For this review, take the finished solid that the model builds, in its own axes (mm). A direction names the side the tool comes from. Give positions to 0.01 mm unless a question says otherwise; leave off trailing zeros. Write each loop counter-clockwise with the first axis right and the second up, starting at its lowest first coordinate (ties: lowest second). Pieces come first, ordered by that corner, then holes.
Q1. Mouldability with a two-part tool opening along X and no side actions: class faces 3 (the cylindrical face through (90.047, -9.33, 29.268)), 4 (the cylindrical face through (140.345, -8.762, 50.263)), 5 (the flat face through (79, -9, 57.15)), 6 (the flat face through (70.353, -9.392, 10.776)) as released by +X, released by -X, zero draft, split by the parting line, or undercut.
Q2. We need section B-B (z = 39.5). Write out the cut boundary in (x, y) (3 decimals), then the cut area to 3 significant figures.
Q3. For line 1 (X direction, y = -9.75, z = 50); line 2 (X direction, y = -11.75, z = 45); line 3 (X direction, y = -13.5, z = 34.5), list the stretches that pass through material, from the lowest coordinate up.
Q4. We need section C-C (x = 95). Write out the cut boundary in (y, z), then the cut area to 3 significant figures.
Q5. We need section D-D (x = 125). Write out the cut boundary in (y, z).
Q6. We need section A-A (x = 50.8). Write out the cut boundary in (y, z) (3 decimals).
Q7. Insertion check: P1, Ø10, axis at x = 137.922, y = -9.525, coming from the -Z side; P2, Ø10, axis at x = 94.5, y = -11.5, coming from the -Z side; P3, Ø6, axis at x = 94.488, y = -9.525, coming from the -Z side. Each pin has a flat end and moves straight along its axis. Give the tip position at first contact, or say it passes through.
Q8. Machinability: for faces 1 (the cylindrical face through (133.48, -9.33, 39.6)), 2 (the flat face through (120.365, -9.392, 28.061)), which of the approach directions +Z, -Z, +X, -X, +Y, -Y give a long, thin tool a straight path to every point of the face, cutting with its end or side? Answer none if there is none.
```python
from build123d import *

# Parameters (mm, degrees)
F1_DEPTH  = 19.05
F2_R      = 2.54
F3_DEPTH  = 50.801
F4_START  = -13.97
F2_R_2    = 4.445
F4_DEPTH  = 40.386
F6_DEPTH  = 10.16
F8_DEPTH  = 10.16
F10_DEPTH = 10.16


with BuildPart() as f1:
    # F0 (on Front) → F1 (new body)
    with BuildSketch(Plane.XZ):
        Polygon((149.77654996, 57.15), (6.35, 57.15), (6.35, 6.35), (49.53, 6.35), (91.7664133997, 15.3276268095), (149.77654996, 41.1554036448), align=None)
    extrude(amount=F1_DEPTH)

    # F2 (on face) → F3 (cut, through all)
    with BuildSketch(Plane.XY.offset(57.15)):
        with Locations((50.8, -9.525)):
            Circle(F2_R)
        with Locations((94.488, -9.525)):
            Circle(F2_R)
        with Locations((137.922, -9.525)):
            Circle(F2_R)
    extrude(amount=-F3_DEPTH, mode=Mode.SUBTRACT)

    # F2 (on face) → F4 (cut)
    with BuildSketch(Plane.XY.offset(57.15).offset(F4_START)):
        with Locations((50.8, -9.525)):
            Circle(F2_R_2)
        with Locations((50.8, -9.525)):
            Circle(F2_R, mode=Mode.SUBTRACT)
        with Locations((94.488, -9.525)):
            Circle(F2_R_2)
        with Locations((94.488, -9.525)):
            Circle(F2_R, mode=Mode.SUBTRACT)
        with Locations((137.922, -9.525)):
            Circle(F2_R_2)
        with Locations((137.922, -9.525)):
            Circle(F2_R, mode=Mode.SUBTRACT)
    extrude(amount=-F4_DEPTH, mode=Mode.SUBTRACT)

    # F5 (on face) → F6 (cut)
    with BuildSketch(Plane(origin=(0, 0, 6.35), x_dir=(1, 0, 0), z_dir=(0, 0, -1))):
        with BuildLine():
            ThreePointArc((21.0968814449, 14.0652501177), (20.97463405, 14.5484294642), (20.6373100259, 14.915334369))
            ThreePointArc((20.6373100259, 14.915334369), (20.0808814449, 14.0652501177), (19.6229011784, 13.1583267056))
            ThreePointArc((19.6229011784, 13.1583267056), (20.6133042324, 13.1999282265), (21.0968814449, 14.0652501177))
        make_face()
        with BuildLine():
            ThreePointArc((19.6229011784, 13.1583267056), (20.0808814449, 14.0652501177), (20.6373100259, 14.915334369))
            ThreePointArc((20.6373100259, 14.915334369), (19.2009996347, 14.5732501177), (19.6229011784, 13.1583267056))
        make_face()
        with BuildLine():
            ThreePointArc((36.8247688031, 4.9847501177), (36.6740906943, 5.5171729052), (36.2667490696, 5.8916735299))
            ThreePointArc((36.2667490696, 5.8916735299), (35.8087688031, 4.9847501177), (35.2523402221, 4.1346658664))
            ThreePointArc((35.2523402221, 4.1346658664), (36.2919481496, 4.0909975126), (36.8247688031, 4.9847501177))
        make_face()
        with BuildLine():
            ThreePointArc((35.2523402221, 4.1346658664), (35.8087688031, 4.9847501177), (36.2667490696, 5.8916735299))
            ThreePointArc((36.2667490696, 5.8916735299), (34.9288869928, 5.4927501177), (35.2523402221, 4.1346658664))
        make_face()
    extrude(amount=-F6_DEPTH, mode=Mode.SUBTRACT)

    # F7 (on face) → F8 (cut)
    with BuildSketch(Plane(origin=(0.8496578997, 0, -3.9973261378), x_dir=(0.9781476007, 0, 0.2079116908), z_dir=(0.2079116908, 0, -0.9781476007))):
        with BuildLine():
            ThreePointArc((64.5139077337, 14.0652501177), (64.3916603388, 14.5484294642), (64.0543363147, 14.915334369))
            ThreePointArc((64.0543363147, 14.915334369), (63.4979077337, 14.0652501177), (63.0399274672, 13.1583267056))
            ThreePointArc((63.0399274672, 13.1583267056), (64.0303305212, 13.1999282265), (64.5139077337, 14.0652501177))
        make_face()
        with BuildLine():
            ThreePointArc((63.0399274672, 13.1583267056), (63.4979077337, 14.0652501177), (64.0543363147, 14.915334369))
            ThreePointArc((64.0543363147, 14.915334369), (62.6180259235, 14.5732501177), (63.0399274672, 13.1583267056))
        make_face()
        with BuildLine():
            ThreePointArc((80.2417950919, 4.9847501177), (80.0911169831, 5.5171729052), (79.6837753584, 5.8916735299))
            ThreePointArc((79.6837753584, 5.8916735299), (79.2257950919, 4.9847501177), (78.6693665109, 4.1346658664))
            ThreePointArc((78.6693665109, 4.1346658664), (79.7089744384, 4.0909975126), (80.2417950919, 4.9847501177))
        make_face()
        with BuildLine():
            ThreePointArc((78.6693665109, 4.1346658664), (79.2257950919, 4.9847501177), (79.6837753584, 5.8916735299))
            ThreePointArc((79.6837753584, 5.8916735299), (78.3459132816, 5.4927501177), (78.6693665109, 4.1346658664))
        make_face()
    extrude(amount=-F8_DEPTH, mode=Mode.SUBTRACT)

    # F9 (on face) → F10 (cut)
    with BuildSketch(Plane(origin=(9.4860255039, 0, -21.30596212), x_dir=(0.9135454576, 0, 0.4067366431), z_dir=(0.4067366431, 0, -0.9135454576))):
        with BuildLine():
            ThreePointArc((105.3219744595, 14.06525), (105.1997270646, 14.5484293465), (104.8624030404, 14.9153342513))
            ThreePointArc((104.8624030404, 14.9153342513), (104.3059744595, 14.06525), (103.847994193, 13.1583265879))
            ThreePointArc((103.847994193, 13.1583265879), (104.8383972469, 13.1999281088), (105.3219744595, 14.06525))
        make_face()
        with BuildLine():
            ThreePointArc((103.847994193, 13.1583265879), (104.3059744595, 14.06525), (104.8624030404, 14.9153342513))
            ThreePointArc((104.8624030404, 14.9153342513), (103.4260926492, 14.57325), (103.847994193, 13.1583265879))
        make_face()
        with BuildLine():
            ThreePointArc((121.0498618176, 4.98475), (120.8991837088, 5.5171727875), (120.4918420841, 5.8916734121))
            ThreePointArc((120.4918420841, 5.8916734121), (120.0338618176, 4.98475), (119.4774332367, 4.1346657487))
            ThreePointArc((119.4774332367, 4.1346657487), (120.5170411641, 4.0909973949), (121.0498618176, 4.98475))
        make_face()
        with BuildLine():
            ThreePointArc((119.4774332367, 4.1346657487), (120.0338618176, 4.98475), (120.4918420841, 5.8916734121))
            ThreePointArc((120.4918420841, 5.8916734121), (119.1539800074, 5.49275), (119.4774332367, 4.1346657487))
        make_face()
    extrude(amount=-F10_DEPTH, mode=Mode.SUBTRACT)


solid = f1.part
```
Computed:
1. face 3: undercut
1. face 4: undercut
1. face 5: zero draft
1. face 6: released by +X
2. outline: (6.35, -19.05) - (146.058, -19.05) - (146.058, 0) - (6.35, 0) - close; hole circle Ø8.89 at (50.8, -9.525); hole circle Ø8.89 at (94.488, -9.525); hole circle Ø8.89 at (137.922, -9.525)
2. area: 2,480 mm2
3. line 1: x = 6.35 to 48.27, 53.33 to 91.96, 97.02 to 135.39, 140.45 to 149.78
3. line 2: x = 6.35 to 49.57, 52.03 to 93.26, 95.71 to 136.7, 139.15 to 149.78
3. line 3: x = 6.35 to 48.81, 52.79 to 92.5, 96.48 to 134.83
4. outline: (-19.05, 16.77) - (-13.94, 16.77) - (-13.94, 43.18) - (-12.01, 43.18) - (-12.01, 57.15) - (-19.05, 57.15) - close; (-7.04, 43.18) - (-5.11, 43.18) - (-5.11, 16.77) - (0, 16.77) - (0, 57.15) - (-7.04, 57.15) - close
4. area: 467 mm2
5. outline: (-19.05, 30.12) - (0, 30.12) - (0, 57.15) - (-19.05, 57.15) - close
6. outline: (-19.05, 6.62) - (-13.97, 6.62) - (-13.97, 43.18) - (-12.065, 43.18) - (-12.065, 57.15) - (-19.05, 57.15) - close; (-6.985, 43.18) - (-5.08, 43.18) - (-5.08, 6.62) - (0, 6.62) - (0, 57.15) - (-6.985, 57.15) - close
7. P1: stops at z = 33.65
7. P2: stops at z = 14.85
7. P3: stops at z = 43.18
8. face 1: -Z
8. face 2: -Z, +X, +Y, -Y
